The model under review builds one solid part; all positions refer to its coordinate system, in mm. A direction names the side the tool comes from. Coordinates: 2 decimals unless noted, no trailing zeros. Order: outer loops, then holes, each group sorted by start corner. A loop starts at its lowest first (then second) coordinate and runs counter-clockwise, first axis right, second up. Notation, with made-up numbers: M 27.25,62.5 L 56.25,62.5 A9 ccw 56.25,73.5 Z; hole C 89,80 d6. An arc over 180 degrees is marked long. One line per item, written item: value.
Autodesk Inventor part; units mm, degrees
ref_plane "YZ Plane" through (0, 0, 0) normal (1, 0, 0) x (0, 1, 0)
ref_plane "XZ Plane" through (0, 0, 0) normal (0, 1, 0) x (-1, 0, 0)
ref_plane "XY Plane" through (0, 0, 0) normal (0, 0, 1) x (1, 0, 0)
sketch "Sketch1" plane through (0, 0, 0) normal (0, 0, 1) x (1, 0, 0)
  line L0 (-10, -10) -> (10, -10)
  line L1 (10, -10) -> (10, 10)
  line L2 (10, 10) -> (-10, 10)
  line L3 (-10, 10) -> (-10, -10)
  line L4 (-10, -10) -> (10, 10) construction
  line L5 (10, -10) -> (-10, 10) construction
  line L6 (-20, 15) -> (-20, -32.5)
  line L7 (-20, 15) -> (-7.0096, 22.5)
  line L8 (-20, 15) -> (-5, 15) construction
  line L9 (-7.0096, 22.5) -> (7.0096, 22.5)
  line L10 (7.0096, 22.5) -> (20, 15)
  line L11 (20, 15) -> (20, -32.5)
  circle A0 centre (0, -32.5) radius 20 construction
  arc A1 (-20, -32.5) -> (20, -32.5) centre (0, -32.5) ccw
  point P0 (0, 0)
  point P1 (0, 22.5)
  point P2 (0, 10)
  dimension "d0" = 20
  dimension "d1" = 20
  dimension "d3" = 15
  dimension "d4" = 30
  dimension "d5" = 15
  dimension "d6" = 150
  dimension "d8" = 40
  dimension "d9" = 5
  dimension "d10" = 40
  dimension "d11" = 55
extrude "Extrusion1" add sketch "Sketch1" along normal blind 18
sketch "Sketch2" plane through (0, 0, 18) normal (0, 0, 1) x (1, 0, 0)
  line L0 (-10, -10) -> (-10, 10)
  line L1 (-10, 10) -> (10, 10)
  line L2 (10, 10) -> (10, -10)
  line L3 (10, -10) -> (-10, -10)
  line L4 (-20, 15) -> (-20, -32.5)
  arc A0 (-20, -32.5) -> (20, -32.5) centre (0, -32.5) ccw
  line L5 (20, -32.5) -> (20, 15)
  line L6 (20, 15) -> (7.0096, 22.5)
  line L7 (7.0096, 22.5) -> (-7.0096, 22.5)
  line L8 (-7.0096, 22.5) -> (-20, 15)
  point P0 (0, 0)
extrude "Extrusion2" add sketch "Sketch2" against normal blind 36 contours L0 L1 L2 L3
sketch "Sketch3" plane through (10, -10, 0) normal (1, 0, 0) x (0, 0, -1)
  circle A0 centre (9, 10) radius 3.25
  line L0 (0, 20) -> (18, 20)
  line L1 (0, 0) -> (0, 20)
  point P0 (0, 10)
  point P1 (9, 20)
  point P2 (0, 10)
  dimension "d16" = 6.5
extrude "Extrusion3" cut sketch "Sketch3" against normal through all
sketch "Sketch4" plane through (0, 0, 18) normal (0, 0, 1) x (1, 0, 0)
  circle A0 centre (0, 5) radius 17.5
  line L0 (7.0096, 22.5) -> (-7.0096, 22.5)
  point P0 (0, 0)
  point P1 (0, 22.5)
  dimension "d19" = 35
extrude "Extrusion4" add sketch "Sketch4" along normal blind 564
sketch "Sketch5" plane through (0, 0, 18) normal (0, 0, 1) x (1, 0, 0)
  circle A0 centre (0, -33) radius 19
  circle A1 centre (0, 5) radius 17.5
  point P0 (0, 0)
  dimension "d22" = 38
  dimension "d23" = 38
extrude "Extrusion5" add sketch "Sketch5" along normal blind 80 contours A0
sketch "Sketch6" plane through (0, 5, 582) normal (0, 0, 1) x (1, 0, 0)
  circle A0 centre (0, 0) radius 17.5
  circle A1 centre (0, 0) radius 10
  point P0 (0, -5)
  dimension "d26" = 20
extrude "Extrusion6" add sketch "Sketch6" along normal blind 18 contours A1
sketch "Sketch8" plane through (0, 0, 0) normal (1, 0, 0) x (0, 1, 0)
  line L0 (15, 600) -> (-5, 600)
  line L1 (-5, 582) -> (15, 582)
  circle A0 centre (5, 591) radius 3.25
  line L2 (15, 600) -> (15, 582)
  line L3 (15, 582) -> (15, 600)
  point P0 (0, 0)
  point P1 (15, 591)
  point P2 (5, 582)
  dimension "d29" = 6.5
extrude "Extrusion7" cut sketch "Sketch8" along normal through all both and the other way through all
properties part number "LinearActuator450" material "Steel, Carbon"
(1) For L1, parallel to Y at x = -1.5, z = 591; L2, parallel to Z at x = 0, y = 5; L3, parallel to Y at x = -2, z = -9, list the stretches that pass through material, from the lowest coordinate up.
Geometry results:
L1: y = -4.89 to 1.75, 8.25 to 14.89
L2: z = -18 to 587.75, 594.25 to 600
L3: y = -10 to -3.25, 3.25 to 10
(2) We need section A-A, the plane y = -40.5. State the section outline as (x, z) points, plus the area to 3 significant figures.
Geometry results:
outline: M -18.33,0 L 18.33,0 L 18.33,18 L 17.46,18 L 17.46,98 L -17.46,98 L -17.46,18 L -18.33,18 Z
area: 3,450 mm2
(3) Mouldability with a two-part tool opening along Y and no side actions: class faces 4 (the cylindrical face through (9.237, 8.83, 590.874)), 5 (the cylindrical face through (-4.119, -14.452, 57.44)), 6 (the flat face through (0, 0, -18)) as +Y half, -Y half, draft (parallel to the pull), parting line (faces both ways), or undercut.
Geometry results:
face 4: parting line
face 5: undercut
face 6: draft
(4) Insertion check: pin 1 Ø11.5 at (x, y) = (2.5, -31) entering from +Z; pin 2 Ø1.5 at (x, y) = (-14, -23) entering from -Z; pin 3 Ø5 at (y, z) = (0, -9) entering from +X; pin 4 Ø3 at (y, z) = (5, 263.5) entering from +X. Each pin has a flat end and moves straight along its axis. Give the tip position at first contact, or say it passes through.
Geometry results:
pin 1: stops at z = 98
pin 2: stops at z = 0
pin 3: passes through
pin 4: stops at x = 17.5
(5) We need section B-B, the plane z = 200. State the section outline as (x, y) points, plus the area to 3 significant figures.
Geometry results:
outline: C 0,5 d35
area: 962 mm2
(6) Tool access review of faces 1 (the flat face through (0, -10, -9)), 2 (the flat face through (8, -3, 582)), 3 (the flat face through (0, -33, 98)): name each direction out of +Z, -Z, +X, -X, +Y, -Y from which nothing blocks a thin tool from reaching the whole face with its end or side.
Geometry results:
face 1: -Z, +X, -X, -Y
face 2: +Z
face 3: +Z, +X, -X, -Y
